Geometry: final body of the model. Coordinates: model frame, mm. A direction names the side the tool comes from. Coordinates: 2 decimals unless noted, no trailing zeros. Loops run counter-clockwise (first coordinate to the right, second up) from the corner with the lowest first, then second, coordinate; pieces in that order, holes last. Notation, with made-up numbers: (40, 12.5) -> (67, 12.5) arc R29 cw to (67, 49.5) -> close; hole circle Ø6 at (-32, -23.75). An arc over 180 degrees is marked (long way). One line per item, written item: value. Start each with the question number.
Item 1: Section query C-C on z = 11.5. Return loops of the section in (x, y), then the cut area to 3 significant figures.
Item 2: Section query D-D on z = 34.5. Return loops of the section in (x, y), then the cut area to 3 significant figures.
Item 3: Section query A-A on y = -6. Return loops of the section in (x, z), then the cut area to 3 significant figures.
Item 4: Set-up query: faces 4 (the cylindrical face through (-19.257, 0.76, 22.47)), 5 (the flat face through (-26, 0.3, 13.8)). Return all of +Z, -Z, +X, -X, +Y, -Y with unobstructed straight access to the full face (end or side cutting, diameter ignored); none if empty.
Item 5: Mould query, pull axis Z, two halves, no side actions, for faces 1 (the flat face through (-13, -8, 0)), 2 (the flat face through (-13, -13.5, 1)), 3 (the cylindrical face through (-24.1, 0.8, 31.9)). Classes: +Z half, -Z half, draft (parallel to the pull), parting line (faces both ways), or undercut.
Item 6: Section query B-B on x = -13. Return loops of the section in (y, z).
Item 7: Ray query, probe 1 along X at (y, z) = (1, 32.5); probe 2 along Z at (x, y) = (-11.5, -4); probe 3 along Z at (x, y) = (-23.5, 0.3). Return the intervals inside material, ascending. Write a range as from..to.
Item 8: Contact query for flat-ended pins moving along their axis: pin 1 Ø13 at (x, z) = (-14.5, 27.5) entering from -Y; pin 2 Ø1.6 at (x, y) = (-15, 1) entering from +Z; pin 3 Ø6 at (x, y) = (-12, -7) entering from +Z. Output: stop coordinate, or through.
Autodesk Inventor part; units mm, degrees
ref_plane "YZ Plane" through (0, 0, 0) normal (1, 0, 0) x (0, 1, 0)
ref_plane "XZ Plane" through (0, 0, 0) normal (0, 1, 0) x (-1, 0, 0)
ref_plane "XY Plane" through (0, 0, 0) normal (0, 0, 1) x (1, 0, 0)
sketch "スケッチ1" plane through (0, 0, 0) normal (0, 1, 0) x (-1, 0, 0)
  line L0 (26, 0) -> (0, 0)
  line L1 (0, 0) -> (0, -89.5474)
  line L2 (0, -89.5474) -> (26, -89.5474)
  line L3 (26, -89.5474) -> (26, 0)
  line L4 (26, 0) -> (0, 0)
  line L5 (0, 0) -> (0, 70)
  line L6 (0, 70) -> (26, 70)
  line L7 (26, 70) -> (26, 0)
  line L8 (26, 32.5) -> (0, 32.5)
  circle A0 centre (13, 32.5) radius 6.25
  circle A1 centre (13, 32.5) radius 13
  point P0 (26, 32.5)
  point P1 (0, 32.5)
  dimension "d2" = 70
  dimension "d3" = 26
  dimension "d4" = 32.5
  dimension "d5" = 12.5
extrude "プレート1" add sketch "スケッチ1" along normal blind 1.5 contours L0 L5 A1 L7 | A1 L8 A0 | L8 A0 A1
sketch "スケッチ3" plane through (0, 1.5, 0) normal (0, 1, 0) x (1, 0, 0)
  circle A0 centre (-23.5, -32.5) radius 0.85
  circle A1 centre (-23.5, -11.5) radius 0.85
  circle A2 centre (-2.5, -11.5) radius 0.85
  circle A3 centre (-2.5, -32.5) radius 0.85
  point P0 (0, 0)
extrude "切り取り1" cut sketch "スケッチ3" against normal blind 1.5
sketch "スケッチ4" plane through (0, 1.5, 1.5) normal (0, 0, -1) x (-1, 0, 0)
  line L0 (26, 0) -> (0, 0)
  line L1 (0, 0) -> (0, -15)
  line L2 (0, -15) -> (26, -15)
  line L3 (26, -15) -> (26, 0)
edge flange "フランジ2" height 15 angle 90 thickness 1.5 bend radius 1.5 thickness toward (0, 0, -1) relief tear relief width 1.5 relief depth 0.75 edges at (-13, 0, 0) wall of the first edge with corners at (-26, 1.5, 1.5) (0, 1.5, 1.5) (0, -13.5, 1.5) (-26, -13.5, 1.5)
bend "曲げ2"
corner "コーナー2"
sketch "スケッチ5" plane through (0, -13.5, 0) normal (0, 0, -1) x (-1, 0, 0)
  line L0 (0, 0) -> (26, 0)
  line L1 (26, 0) -> (26, 15)
  line L2 (26, 15) -> (0, 15)
  line L3 (0, 15) -> (0, 0)
  line L4 (26, 12) -> (26, 0)
  line L5 (0, 0) -> (0, 12)
  line L6 (0, 15) -> (26, 0)
  line L7 (26, 15) -> (0, 0)
  line L8 (4, 12.6923) -> (22, 12.6923)
  line L9 (22, 12.6923) -> (22, 2.3077)
  line L10 (22, 2.3077) -> (4, 2.3077)
  line L11 (4, 2.3077) -> (4, 12.6923)
  circle A0 centre (4, 12.6923) radius 0.8
  circle A1 centre (22, 12.6923) radius 0.8
  circle A2 centre (4, 2.3077) radius 0.8
  circle A3 centre (22, 2.3077) radius 0.8
  circle A4 centre (13, 7.5) radius 0.8
  point P0 (0, 13.5)
  dimension "d35" = 15
  dimension "d36" = 4
  dimension "d37" = 1.6
  dimension "d38" = 1.6
  dimension "d39" = 1.6
  dimension "d40" = 1.6
  dimension "d43" = 1.6
extrude "切り取り3" cut sketch "スケッチ5" against normal blind 1.5 contours A2 L11 L7 | L7 L10 A2 | A3 L10 L6 | L6 L9 A3 | L11 A2 L7 | L7 A2 L10 | L10 A3 L6 | L6 A3 L9 | A4 L6 L7 | L7 L6 A4 | L6 L7 A4 | L6 A4 L7
sketch "スケッチ6" plane through (0, 1.5, 0) normal (0, 1, 0) x (1, 0, 0)
  circle A0 centre (-2.5, -32.5) radius 0.85
  circle A1 centre (-23.5, -32.5) radius 0.85
  circle A2 centre (-23.5, -11.5) radius 0.85
  circle A3 centre (-2.5, -11.5) radius 0.85
  line L0 (-2.5, -32.5) -> (-23.5, -32.5)
  line L1 (-23.5, -32.5) -> (-23.5, -11.5)
  line L2 (-23.5, -11.5) -> (-2.5, -11.5)
  line L3 (-2.5, -11.5) -> (-2.5, -32.5)
  line L4 (-5.5, -32.5) -> (-20.5, -32.5)
  line L5 (-20.5, -20.0376) -> (-20.5, -10)
  line L6 (-17.5, -7) -> (-8.5, -7)
  line L7 (-5.5, -10) -> (-5.5, -20.0376)
  circle A4 centre (-13, -32.5) radius 6.25
  line L8 (0, -3) -> (-26, -3)
  arc A5 (-9.5189, -22.8592) -> (-16.4811, -22.8592) centre (-13, -32.5) ccw
  arc A6 (-23.2186, -31.6979) -> (-23.2186, -33.3021) centre (-13, -32.5) ccw
  arc A7 (-2.7814, -33.3021) -> (-2.7814, -31.6979) centre (-13, -32.5) ccw
  arc A8 (-9.5189, -22.8592) -> (-5.5, -20.0376) centre (-8.5, -20.0376) ccw
  arc A9 (-20.5, -20.0376) -> (-16.4811, -22.8592) centre (-17.5, -20.0376) ccw
  arc A10 (-5.5, -10) -> (-8.5, -7) centre (-8.5, -10) ccw
  arc A11 (-17.5, -7) -> (-20.5, -10) centre (-17.5, -10) ccw
  point P0 (0, 0)
  point P1 (-20.5, -7)
  point P2 (-5.5, -7)
  point P3 (-5.5, -25.5134)
  point P4 (-20.5, -25.5134)
  dimension "d46" = 3
  dimension "d47" = 3
  dimension "d49" = 4
  dimension "d50" = 4
  dimension "d53" = 3
  dimension "d54" = 3
extrude "切り取り4" cut sketch "スケッチ6" against normal blind 1.5 contours L7 A8 A5 A9 L5 L2 | L2 L5 A11 L6 A10 L7
fillet "フィレット1" radius 2 2 edges at (-26, -13.5, 0.75) (0, -13.5, 0.75)
equation "\"d23\" = Thickness"
equation "\"d44\" = Thickness"
equation "\"d51\" = Thickness"
equation "\"d12\" = Thickness"
equation "\"d25\" = BendReliefWidth"
equation "\"d26\" = BendReliefDepth"
equation "\"d27\" = MinimumRemnant"
equation "\"d28\" = TransitionRadius"
equation "\"d31\" = BendRadius"
equation "\"d32\" = CornerReliefSize"
equation "\"d33\" = GapSize"
equation "\"d34\" = JacobiRadiusSize"
equation "\"BendRadius\" = Thickness"
equation "\"BendReliefWidth\" = Thickness"
equation "\"BendReliefDepth\" = 0.5 * Thickness"
equation "\"CornerReliefSize\" = 4 * Thickness"
equation "\"MinimumRemnant\" = 2 * Thickness"
equation "\"TransitionRadius\" = BendRadius"
equation "\"JacobiRadiusSize\" = BendRadius"
equation "\"GapSize\" = Thickness"
properties part number "toe_front" material "アルミニウム 6061"
Reply:
1. outline: (-26, 0) -> (-24.35, 0) -> (-24.35, 1.5) -> (-26, 1.5) -> close; (-22.65, 0) -> (-20.5, 0) -> (-20.5, 1.5) -> (-22.65, 1.5) -> close; (-5.5, 0) -> (-3.35, 0) -> (-3.35, 1.5) -> (-5.5, 1.5) -> close; (-1.65, 0) -> (0, 0) -> (0, 1.5) -> (-1.65, 1.5) -> close
1. area: 11.4 mm²
2. outline: (-25.85, 0) -> (-18.92, 0) -> (-18.92, 1.5) -> (-25.85, 1.5) -> close; (-7.08, 0) -> (-0.15, 0) -> (-0.15, 1.5) -> (-7.08, 1.5) -> close
2. area: 20.8 mm²
3. outline: (-26, 0) -> (-13.8, 0) -> (-13.8, 1.5) -> (-26, 1.5) -> close; (-12.2, 0) -> (0, 0) -> (0, 1.5) -> (-12.2, 1.5) -> close
3. area: 36.6 mm²
4. face 4: +Y, -Y
4. face 5: +Z, -Z, -X, +Y, -Y
5. face 1: -Z half
5. face 2: draft
5. face 3: undercut
6. outline: (-13.5, 0) -> (-6.8, 0) -> (-6.8, 1.5) -> (-13.5, 1.5) -> close; (-5.2, 0) -> (-1.5, 0) arc R3 ccw to (1.5, 3) -> (1.5, 7) -> (0, 7) -> (0, 3) arc R1.5 cw to (-1.5, 1.5) -> (-5.2, 1.5) -> close; (0, 22.25) -> (1.5, 22.25) -> (1.5, 26.25) -> (0, 26.25) -> close; (0, 38.75) -> (1.5, 38.75) -> (1.5, 45.5) -> (0, 45.5) -> close
7. probe 1: x = -26..-24.35, -22.65..-19.25, -6.75..-3.35, -1.65..0
7. probe 2: z = 0..1.5
7. probe 3: z = 0.6..10.65, 12.35..31.65, 33.35..40.16
8. pin 1: stops at y = 0
8. pin 2: stops at z = 45.44
8. pin 3: stops at z = 1.5
